```python
from build123d import *

# Parameters (mm, degrees)
BOSS_EXTRUDE1_DEPTH      = 26
BOSS_EXTRUDE1_2_DEPTH    = 26
BOSS_EXTRUDE1_3_DEPTH    = 26
BOSS_EXTRUDE1_4_DEPTH    = 26
BOSS_EXTRUDE1_5_DEPTH    = 26
BOSS_EXTRUDE1_6_DEPTH    = 26
BOSS_EXTRUDE2_DEPTH      = 0.2
BOSS_EXTRUDE2_DEPTH_BACK = 2
SKETCH2_R                = 9
SKETCH2_R_2              = 7.5
BOSS_EXTRUDE3_DEPTH      = 0.2
BOSS_EXTRUDE3_DEPTH_BACK = 2
SKETCH3_R                = 9
SKETCH3_R_2              = 7.5


with BuildPart() as part:
    # Sketch1 → Boss-Extrude1 (new body)
    with BuildSketch(Plane(origin=(0, 0, 0), x_dir=(0, 0, -1), z_dir=(1, 0, 0))):
        with BuildLine():
            ThreePointArc((-1.809150339, 8.816290323), (-4.5, 7.794228634), (-6.730556217, 5.974915314))
            ThreePointArc((-6.730556217, 5.974915314), (-5.469327251, 5.568079356), (-4.702852692, 4.487000842))
            ThreePointArc((-4.702852692, 4.487000842), (-3.25, 5.629165125), (-1.53443037, 6.316290323))
            ThreePointArc((-1.53443037, 6.316290323), (-2.087434547, 7.520616019), (-1.809150339, 8.816290323))
        make_face()
    extrude(amount=BOSS_EXTRUDE1_DEPTH)



with BuildPart() as body_2:
    # Sketch1 → Boss-Extrude1 2 (new body)
    with BuildSketch(Plane(origin=(0, 0, 0), x_dir=(0, 0, -1), z_dir=(1, 0, 0))):
        with BuildLine():
            ThreePointArc((6.237283062, 1.82928948), (7.556761798, 1.952536663), (8.539706556, 2.841375009))
            ThreePointArc((8.539706556, 2.841375009), (9, 0), (8.539706556, -2.841375009))
            ThreePointArc((8.539706556, -2.841375009), (7.556761798, -1.952536663), (6.237283062, -1.82928948))
            ThreePointArc((6.237283062, -1.82928948), (6.5, 0), (6.237283062, 1.82928948))
        make_face()
    extrude(amount=BOSS_EXTRUDE1_2_DEPTH)


with BuildPart() as body_3:
    # Sketch1 → Boss-Extrude1 3 (new body)
    with BuildSketch(Plane(origin=(0, 0, 0), x_dir=(0, 0, -1), z_dir=(1, 0, 0))):
        with BuildLine():
            ThreePointArc((-1.53443037, -6.316290323), (-2.087434547, -7.520616019), (-1.809150339, -8.816290323))
            ThreePointArc((-1.809150339, -8.816290323), (-4.5, -7.794228634), (-6.730556217, -5.974915314))
            ThreePointArc((-6.730556217, -5.974915314), (-5.469327251, -5.568079356), (-4.702852692, -4.487000842))
            ThreePointArc((-4.702852692, -4.487000842), (-3.25, -5.629165125), (-1.53443037, -6.316290323))
        make_face()
    extrude(amount=BOSS_EXTRUDE1_3_DEPTH)


with BuildPart() as body_4:
    # Sketch1 → Boss-Extrude1 4 (new body)
    with BuildSketch(Plane(origin=(0, 0, 0), x_dir=(0, 0, -1), z_dir=(1, 0, 0))):
        with BuildLine():
            ThreePointArc((1.53443037, 6.316290323), (2.087434547, 7.520616019), (1.809150339, 8.816290323))
            ThreePointArc((1.809150339, 8.816290323), (4.5, 7.794228634), (6.730556217, 5.974915314))
            ThreePointArc((6.730556217, 5.974915314), (5.469327251, 5.568079356), (4.702852692, 4.487000842))
            ThreePointArc((4.702852692, 4.487000842), (3.25, 5.629165125), (1.53443037, 6.316290323))
        make_face()
    extrude(amount=BOSS_EXTRUDE1_4_DEPTH)


with BuildPart() as body_5:
    # Sketch1 → Boss-Extrude1 5 (new body)
    with BuildSketch(Plane(origin=(0, 0, 0), x_dir=(0, 0, -1), z_dir=(1, 0, 0))):
        with BuildLine():
            ThreePointArc((-6.237283062, 1.82928948), (-6.5, 0), (-6.237283062, -1.82928948))
            ThreePointArc((-6.237283062, -1.82928948), (-7.556761798, -1.952536663), (-8.539706556, -2.841375009))
            ThreePointArc((-8.539706556, -2.841375009), (-9, 0), (-8.539706556, 2.841375009))
            ThreePointArc((-8.539706556, 2.841375009), (-7.556761798, 1.952536663), (-6.237283062, 1.82928948))
        make_face()
    extrude(amount=BOSS_EXTRUDE1_5_DEPTH)


with BuildPart() as body_6:
    # Sketch1 → Boss-Extrude1 6 (new body)
    with BuildSketch(Plane(origin=(0, 0, 0), x_dir=(0, 0, -1), z_dir=(1, 0, 0))):
        with BuildLine():
            ThreePointArc((4.702852692, -4.487000842), (5.469327251, -5.568079356), (6.730556217, -5.974915314))
            ThreePointArc((6.730556217, -5.974915314), (4.5, -7.794228634), (1.809150339, -8.816290323))
            ThreePointArc((1.809150339, -8.816290323), (2.087434547, -7.520616019), (1.53443037, -6.316290323))
            ThreePointArc((1.53443037, -6.316290323), (3.25, -5.629165125), (4.702852692, -4.487000842))
        make_face()
    extrude(amount=BOSS_EXTRUDE1_6_DEPTH)


with BuildPart() as part_1:
    add(part.part)

    add(body_2.part)  # Boss-Extrude2 merges body 2

    add(body_3.part)  # Boss-Extrude2 merges body 3

    add(body_4.part)  # Boss-Extrude2 merges body 4

    add(body_5.part)  # Boss-Extrude2 merges body 5

    add(body_6.part)  # Boss-Extrude2 merges body 6
    # Sketch2 → Boss-Extrude2 (add, two sides: drawn at the far end of the back side and taken through both)
    with BuildSketch(Plane(origin=(26, 0, 0), x_dir=(0, 0, -1), z_dir=(1, 0, 0)).offset(-BOSS_EXTRUDE2_DEPTH_BACK)):
        with Locations(Location((0, 0, 0), (0, 0, 161.596419423))):
            Circle(SKETCH2_R)
        with Locations(Location((0, 0, 0), (0, 0, 165.71895949))):
            Circle(SKETCH2_R_2, mode=Mode.SUBTRACT)
    extrude(amount=BOSS_EXTRUDE2_DEPTH + BOSS_EXTRUDE2_DEPTH_BACK)

    # Sketch3 → Boss-Extrude3 (add, two sides: drawn at the far end of the back side and taken through both)
    with BuildSketch(Plane.ZY.offset(-BOSS_EXTRUDE3_DEPTH_BACK)):
        Circle(SKETCH3_R)
        with Locations(Location((0, 0, 0), (0, 0, 14.28104051))):
            Circle(SKETCH3_R_2, mode=Mode.SUBTRACT)
    extrude(amount=BOSS_EXTRUDE3_DEPTH + BOSS_EXTRUDE3_DEPTH_BACK)


solid = part_1.part
```
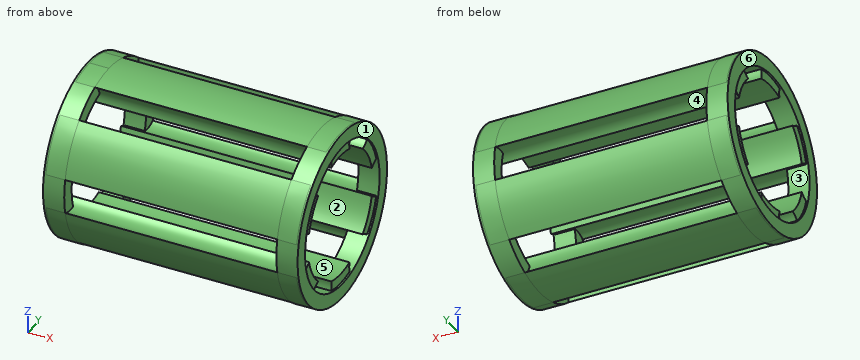
Can you work these out from the model? Positions are in its coordinate system, mm. Face numbers are marked on the shaded views. A direction names the side the tool comes from. Coordinates: 2 decimals unless noted, no trailing zeros. Order: outer loops, then holes, each group sorted by start corner. A loop starts at its lowest first (then second) coordinate and runs counter-clockwise, first axis right, second up.
1. If we section it at B-B (z = 0): Please give me the cut outline in (x, y), then the cut area to 3 significant figures.
2. Thinking about a two-plate mould opening in Z: for the marked faces 1, 2 and 3, which applies, +Z half, -Z half, draft (parallel to the pull), parting line (faces both ways), or undercut?
3. For the marked faces 4, 5 and 6, which set-ups out of +Z, -Z, +X, -X, +Y, -Y let a thin tool reach every point of the face, with its end or its side?
4. If we section it at D-D (z = 3): Please give me the cut outline in (x, y).
5. If we section it at A-A (x = 22.5): Please give me the cut outline in (y, z) (3 decimals), then the cut area to 3 significant figures.
6. I'm going to push flat-ended pins straight in: pin 1 (0.8 mm diameter, centred on y = -5.5, z = 3, fed in from -X); pin 2 (2 mm diameter, centred on x = 21.5, y = -1.5, fed in from -Z); pin 3 (0.8 mm diameter, centred on y = -5.5, z = 3.5, fed in from +X); pin 4 (9 mm diameter, centred on y = 0, z = 0, fed in from -X). Where does each tip first touch, or does it pass through?
7. If we section it at C-C (y = -3.25): Please give me the cut outline in (x, z).
8. I need wall thicknesses on line 1 (Y direction, x = 25.45, z = 0); line 2 (X direction, y = -3, z = -8); line 3 (Z direction, x = 12, y = 2). Which ranges of each line are inside material? Lowest first, please.
Entries:
1. outline: (-0.2, -9) - (2, -9) - (2, -7.5) - (-0.2, -7.5) - close; (-0.2, 7.5) - (2, 7.5) - (2, 9) - (-0.2, 9) - close; (24, -9) - (26.2, -9) - (26.2, -7.5) - (24, -7.5) - close; (24, 7.5) - (26.2, 7.5) - (26.2, 9) - (24, 9) - close
1. area: 13.2 mm2
2. face 1: draft
2. face 2: undercut
2. face 3: undercut
3. face 4: none
3. face 5: +X, -X
3. face 6: +Z, -Z, -X, +Y, -Y
4. outline: (-0.2, -8.49) - (26.2, -8.49) - (26.2, -6.87) - (26, -6.87) - (26, -5.77) - (0, -5.77) - (0, -6.87) - (-0.2, -6.87) - close; (-0.2, 6.87) - (0, 6.87) - (0, 5.77) - (26, 5.77) - (26, 6.87) - (26.2, 6.87) - (26.2, 8.49) - (-0.2, 8.49) - close
5. outline: (-8.816, -1.809) arc R9 ccw to (-5.975, -6.731) arc R2.1 cw to (-4.487, -4.703) arc R6.5 cw to (-6.316, -1.534) arc R2.1 cw to start; (-8.816, 1.809) arc R2.1 cw to (-6.316, 1.534) arc R6.5 cw to (-4.487, 4.703) arc R2.1 cw to (-5.975, 6.731) arc R9 ccw to start; (-2.841, -8.54) arc R9 ccw to (2.841, -8.54) arc R2.1 cw to (1.829, -6.237) arc R6.5 cw to (-1.829, -6.237) arc R2.1 cw to start; (-2.841, 8.54) arc R2.1 cw to (-1.829, 6.237) arc R6.5 cw to (1.829, 6.237) arc R2.1 cw to (2.841, 8.54) arc R9 ccw to start; (4.487, -4.703) arc R2.1 cw to (5.975, -6.731) arc R9 ccw to (8.816, -1.809) arc R2.1 cw to (6.316, -1.534) arc R6.5 cw to start; (4.487, 4.703) arc R6.5 cw to (6.316, 1.534) arc R2.1 cw to (8.816, 1.809) arc R9 ccw to (5.975, 6.731) arc R2.1 cw to start
5. area: 62.6 mm2
6. pin 1: stops at x = 0
6. pin 2: stops at z = -8.99
6. pin 3: stops at x = 26
6. pin 4: passes through
7. outline: (-0.2, -8.39) - (2, -8.39) - (2, -6.76) - (-0.2, -6.76) - close; (-0.2, 6.76) - (2, 6.76) - (2, 8.39) - (-0.2, 8.39) - close; (24, -8.39) - (26.2, -8.39) - (26.2, -6.76) - (24, -6.76) - close; (24, 6.76) - (26.2, 6.76) - (26.2, 8.39) - (24, 8.39) - close
8. line 1: y = -9 to -7.5, 7.5 to 9
8. line 2: x = -0.2 to 2, 24 to 26.2
8. line 3: z = -8.77 to -7.66, 7.66 to 8.77
